Job drawing, mm, ordinate dimensions from the low corner. One solid piece. A direction names the side the tool comes from. Round coordinates to 2 decimals unless told otherwise and drop trailing zeros. Order: outer loops, then holes, each group sorted by start corner. A loop starts at its lowest first (then second) coordinate and runs counter-clockwise, first axis right, second up. Notation, with made-up numbers: (-35.75, 48.5) - (-3.75, 48.5) arc R19 ccw to (-3.75, 79.5) - close; hole circle Ø10 at (46.25, 3). An arc over 180 degrees is marked (long way). Write each question's results on one line, items separated by ' | '. Start each with the question number.
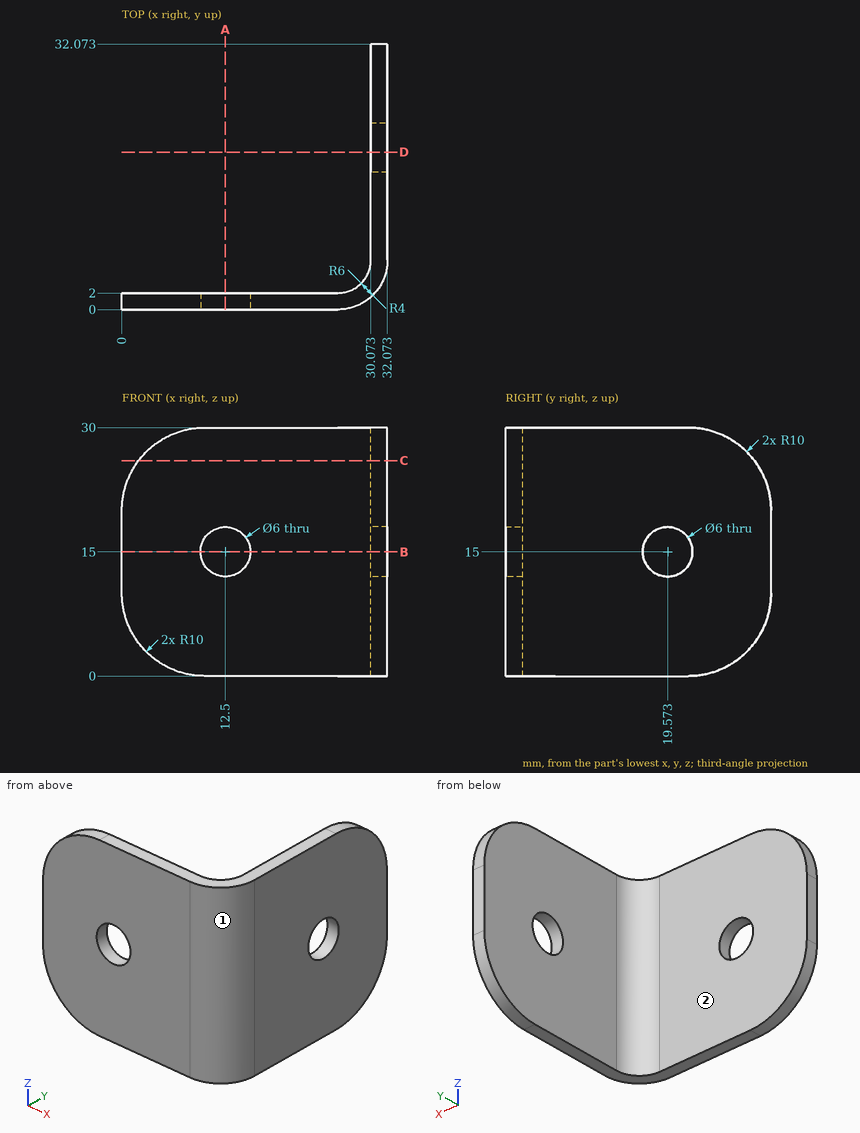
1. Cut at A-A (x = 12.5). List the corners of the cut face in (y, z).
2. Cut at D-D (y = 19). List the corners of the cut face in (x, z).
3. Cut at C-C (z = 26). List the corners of the cut face in (x, y).
4. Flat gauge pins, fed straight in: pin 1 Ø8 at (x, z) = (13.5, 21) entering from +Y; pin 2 Ø6 at (y, z) = (18, 20) entering from -X. Where does each tip first touch, or does it go through?
5. Cut at B-B (z = 15). List the corners of the cut face in (x, y), plus the area to 3 significant figures.
6. 3-axis set-ups, long thin cutter, end or side, ignore diameter. For the marked faces 1 and 2: which of +Z, -Z, +X, -X, +Y, -Y reach the whole face in a straight line?
7. Wall check: line 1 (X direction, y = 28.5, z = 12); line 2 (Y direction, x = 26, z = 20); line 3 (X direction, y = 1.4, z = 15). Give the ranges that are in metal, low to high. Write a range as from..to.
A:
1) outline: (0, 0) - (2, 0) - (2, 12) - (0, 12) - close; (0, 18) - (2, 18) - (2, 30) - (0, 30) - close
2) outline: (30.07, 0) - (32.07, 0) - (32.07, 12.06) - (30.07, 12.06) - close; (30.07, 17.94) - (32.07, 17.94) - (32.07, 30) - (30.07, 30) - close
3) outline: (2, 0) - (26.07, 0) arc R6 ccw to (32.07, 6) - (32.07, 30.07) - (30.07, 30.07) - (30.07, 6) arc R4 cw to (26.07, 2) - (2, 2) - close
4) pin 1: stops at y = 2 | pin 2: stops at x = 30.07
5) outline: (0, 0) - (9.5, 0) - (9.5, 2) - (0, 2) - close; (15.5, 0) - (26.07, 0) arc R6 ccw to (32.07, 6) - (32.07, 16.57) - (30.07, 16.57) - (30.07, 6) arc R4 cw to (26.07, 2) - (15.5, 2) - close; (30.07, 22.57) - (32.07, 22.57) - (32.07, 32.07) - (30.07, 32.07) - close | area: 96.0 mm^2
6) face 1: +Z, -Z, +X, -Y | face 2: +Z, -Z, -X, +Y
7) line 1: x = 30.07..32.07 | line 2: y = 0..2 | line 3: x = 0..9.5, 15.5..29.93
